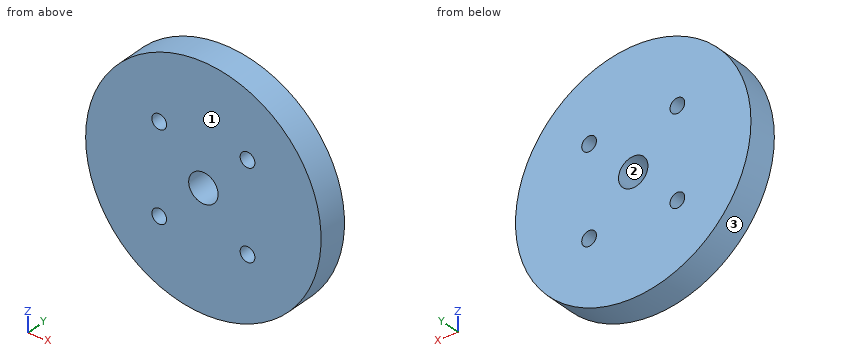
Autodesk Inventor part; units mm, degrees
ref_plane "YZ Plane" through (0, 0, 0) normal (1, 0, 0) x (0, 1, 0)
ref_plane "XZ Plane" through (0, 0, 0) normal (0, 1, 0) x (-1, 0, 0)
ref_plane "XY Plane" through (0, 0, 0) normal (0, 0, 1) x (1, 0, 0)
sketch "Block1" plane through (0, 0, 0) normal (0, 0, 1) x (1, 0, 0)
  circle A0 centre (0, 0) radius 60.22
  circle A1 centre (-30, -30) radius 2.72
  circle A2 centre (30, -30) radius 2.72
  circle A3 centre (0, 0) radius 5.22
  circle A4 centre (-30, 30) radius 2.72
  circle A5 centre (30, 30) radius 2.72
sketch "Block2" plane through (0, 0, 0) normal (0, 0, 1) x (1, 0, 0)
  circle A0 centre (0, 0) radius 40.22
  circle A1 centre (20, 20) radius 2.72
  circle A2 centre (-20, 20) radius 2.72
  circle A3 centre (0, 0) radius 5.22
  circle A4 centre (20, -20) radius 2.72
  circle A5 centre (-20, -20) radius 2.72
sketch "Block3" plane through (0, 0, 0) normal (0, 0, 1) x (1, 0, 0)
  circle A0 centre (0, 0) radius 40.22
  circle A1 centre (15, -15) radius 2.72
  circle A2 centre (-15, -15) radius 2.72
  circle A3 centre (0, 0) radius 5.22
  circle A4 centre (15, 15) radius 2.72
  circle A5 centre (-15, 15) radius 2.72
sketch "Sketch1" plane through (0, 0, 0) normal (0, 1, 0) x (-1, 0, 0)
  circle A0 centre (0, 0) radius 40
  circle A1 centre (0, 0) radius 5
  circle A2 centre (15, 15) radius 2.5
  line L0 (56.308, 0) -> (-56.308, 0)
  line L1 (0, -56.308) -> (0, 56.308)
  circle A3 centre (15, -15) radius 2.5
  circle A4 centre (-15, 15) radius 2.5
  circle A5 centre (-15, -15) radius 2.5
  dimension "d0" = 80
  dimension "d3" = 10
  dimension "d6" = 5
  dimension "d7" = 15
  dimension "d8" = 15
extrude "Extrusion3" add sketch "Sketch1" along normal blind 10 contours L0 A1 L1 A0 | A0 L1 A1 L0 | L1 A1 L0 A0 | A0 L0 A1 L1
sketch "Sketch6" plane through (0, 0, 0) normal (0, -1, 0) x (1, 0, 0)
  circle A0 centre (0, 0) radius 5
  circle A1 centre (15, 15) radius 2.5
  circle A2 centre (15, -15) radius 2.5
  circle A3 centre (-15, -15) radius 2.5
  circle A4 centre (-15, 15) radius 2.5
  circle A5 centre (0, 0) radius 40
sketch "DXF" plane through (0, 0, 0) normal (0, 1, 0) x (-1, 0, 0)
  point P0 (0, 0)
properties part number "drivepullySide"
For this review, take the finished solid that the model builds, in its own axes (mm). Face numbers are marked on the shaded views. Give positions to 0.01 mm unless a question says otherwise; leave off trailing zeros. Write each loop counter-clockwise with the first axis right and the second up, starting at its lowest first coordinate (ties: lowest second). Pieces come first, ordered by that corner, then holes. Notation, with made-up numbers: M 7,29 L 58,29 A31 ccw 58,67 Z; hole C 37.5,81.25 d3. An arc over 180 degrees is marked long. Answer as CSV lines item,"result".
1. For pin 1 (5 mm diameter, centred on y = 2.5, z = -8.5, fed in from -X); pin 2 (1.5 mm diameter, centred on y = 5, z = 11.5, fed in from +X); pin 3 (6 mm diameter, centred on x = -2, y = 3.5, fed in from +Z), all flat-tipped, find the tip position at first contact; note any pin that passes through.
Findings:
pin 1,"stops at x = -39.55"
pin 2,"stops at x = 38.53"
pin 3,"stops at z = 40"
2. Wall thickness on line 1 (X direction, y = 9.5, z = -13.5); line 2 (Z direction, x = 15, y = 2.75); line 3 (X direction, y = 8.25, z = 16): over which ranges is each line inside the solid? List them lowest first.
Findings:
line 1,"x = -37.65 to -17, -13 to 13, 17 to 37.65"
line 2,"z = -37.08 to -17.5, -12.5 to 12.5, 17.5 to 37.08"
line 3,"x = -36.66 to -17.29, -12.71 to 12.71, 17.29 to 36.66"
3. Draft analysis for pull direction Z (two halves, no side actions). For the marked faces 1, 2 and 3, state which applies: +Z half, -Z half, draft (parallel to the pull), parting line (faces both ways), or undercut.
Findings:
face 1,"draft"
face 2,"undercut"
face 3,"parting line"
4. Consider section D-D, the plane x = 15. Write out the cut boundary in (y, z).
Findings:
outline,"M 0,-37.08 L 10,-37.08 L 10,-17.5 L 0,-17.5 Z; M 0,-12.5 L 10,-12.5 L 10,12.5 L 0,12.5 Z; M 0,17.5 L 10,17.5 L 10,37.08 L 0,37.08 Z"
5. Consider section A-A, the plane z = 0. Write out the cut boundary in (x, y).
Findings:
outline,"M -40,0 L -5,0 L -5,10 L -40,10 Z; M 5,0 L 40,0 L 40,10 L 5,10 Z"
6. Consider section C-C, the plane z = -13.5. Write out the cut boundary in (x, y).
Findings:
outline,"M -37.65,0 L -17,0 L -17,10 L -37.65,10 Z; M -13,0 L 13,0 L 13,10 L -13,10 Z; M 17,0 L 37.65,0 L 37.65,10 L 17,10 Z"
7. Consider section B-B, the plane x = 0. Write out the cut boundary in (y, z), then the cut area to 3 significant figures.
Findings:
outline,"M 0,-40 L 10,-40 L 10,-5 L 0,-5 Z; M 0,5 L 10,5 L 10,40 L 0,40 Z"
area,"700 mm2"
